Geometry check sheet. Reference: the model listing, model coordinates, mm. Face numbers are marked on the shaded views. A direction names the side the tool comes from. Round coordinates to 2 decimals unless told otherwise and drop trailing zeros. Order: outer loops, then holes, each group sorted by start corner. A loop starts at its lowest first (then second) coordinate and runs counter-clockwise, first axis right, second up. Notation, with made-up numbers: M 17,39 L 72,39 A26 ccw 72,68 Z; hole C 33.25,49.25 d2. An arc over 180 degrees is marked long. Answer as a JSON object with one key per item and string values. Group by question number.
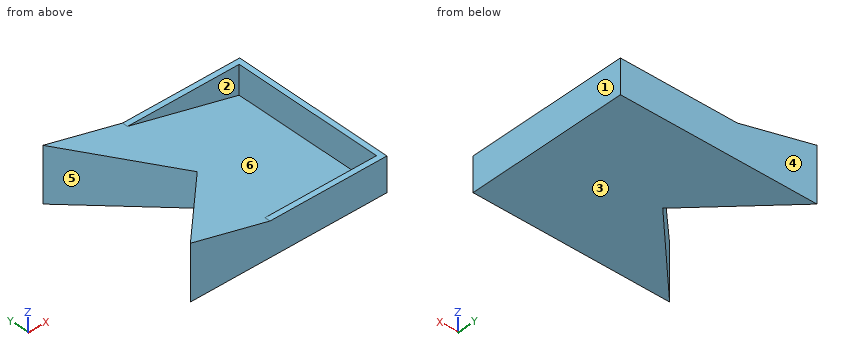
```python
from build123d import *

# Parameters (mm, degrees)
F3_DEPTH  = 59
F4_W      = 59
F4_H      = 12.5
F5_DEPTH  = 2
F6_W      = 65
F6_H      = 12.5
F7_DEPTH  = 2
F8_W      = 65
F8_H      = 12.5
F9_DEPTH  = 2
F11_DEPTH = 25


with BuildPart() as f3:
    # F2 (on offset) → F3 (new body)
    with BuildSketch(Plane.XZ.offset(59)):
        Polygon((0, 20), (0, 0), (70, 0), (70, 2), align=None)
    extrude(amount=-F3_DEPTH)

    # F4 (on offset) → F5 (join)
    with BuildSketch(Plane.YZ.offset(72)):
        with Locations((-29.5, 6.25)):
            Rectangle(F4_W, F4_H)
    extrude(amount=-F5_DEPTH)

    # F6 (on Front) → F7 (join)
    with BuildSketch(Plane.XZ):
        with Locations((39.109939, 6.25)):
            Rectangle(F6_W, F6_H)
    extrude(amount=F7_DEPTH)

    # F8 (on offset) → F9 (join)
    with BuildSketch(Plane.XZ.offset(59)):
        with Locations((39.260793, 6.25)):
            Rectangle(F8_W, F8_H)
    extrude(amount=-F9_DEPTH)

    # F10 (on Top) → F11 (cut)
    with BuildSketch(Plane.XY):
        Polygon((29.5, -29.5), (0, 0), (0, -59), align=None)
    extrude(amount=F11_DEPTH, mode=Mode.SUBTRACT)


solid = f3.part
```
1) Sectioned sample at C-C (y = -45). Record the boundary of the cut face in (x, z).
2) Sectioned sample at D-D (z = 16). Record the boundary of the cut face in (x, y).
3) Release check for a two-part mould opening along X. For the marked faces 1, 2 and 3 record: +X half, -X half, draft (parallel to the pull), parting line (faces both ways), or undercut.
4) Set-up check for the marked faces 4, 5 and 6: record each of +Z, -Z, +X, -X, +Y, -Y from which the full face is reachable in a straight line by a thin tool's end or side.
5) Sectioned sample at A-A (x = 56). Record the boundary of the cut face in (y, z).
6) Thickness scan on line 1 along Y through (x, z) = (45.5, 9.25); line 2 along Y through (x, z) = (22, 9.25); line 3 along Z through (x, y) = (56, -14). Record the ranges inside material, lowest first. Write a range as [from, to].
7) Go/stop test with flat-tipped pins: P1, Ø13, axis at x = 44, y = -41, coming from the +Z side; P2, Ø5, axis at y = -31.5, z = 7, coming from the -X side; P3, Ø1.5, axis at x = 29.5, y = -25, coming from the +Z side. Record where each tip stops, or that it passes through.
8) Sectioned sample at B-B (z = 3.5). Record the boundary of the cut face in (x, y).
Final values:
{
 "1": {"outline": "M 14,0 L 72,0 L 72,12.5 L 70,12.5 L 70,2 L 14,16.4 Z"},
 "2": {"outline": "M 0,-59 L 15.56,-59 L 15.56,-43.44 Z; M 0,0 L 15.56,-15.56 L 15.56,0 Z"},
 "3": {"face 1": "+X half", "face 2": "undercut", "face 3": "draft"},
 "4": {"face 4": "+Z, -Z, +X, -X, +Y", "face 5": "+Z, -Z, -X", "face 6": "+Z"},
 "5": {"outline": "M -59,0 L 0,0 L 0,12.5 L -2,12.5 L -2,5.6 L -57,5.6 L -57,12.5 L -59,12.5 Z"},
 "6": {"line 1": "y = [-59, -57], [-2, 0]", "line 2": "y = [-59, -37], [-22, 0]", "line 3": "z = [0, 5.6]"},
 "7": {"P1": "stops at z = 10.36", "P2": "stops at x = 25", "P3": "stops at z = 12.61"},
 "8": {"outline": "M 0,-59 L 72,-59 L 72,0 L 0,0 L 29.5,-29.5 Z; hole M 64.17,-57 L 70,-57 L 70,-2 L 64.17,-2 Z"}
}
